For this review, use the dimensioned drawing (mm, ordinates from the lowest corner) and the shaded views. A direction names the side the tool comes from. Give positions to 0.01 mm unless a question says otherwise; leave off trailing zeros. Order: outer loops, then holes, each group sorted by start corner. A loop starts at its lowest first (then second) coordinate and runs counter-clockwise, first axis right, second up. Notation, with made-up numbers: M -24,-30.5 L 3,-30.5 A24 ccw 3,5.5 Z; hole C -27,0.25 d5. An arc over 180 degrees is marked long. Use CSV: the item, a comma, the result in double quotes. Start each with the question number.
(1) Consider section C-C (x = 21). Write out the cut boundary in (y, z).
(2) Consider section B-B (y = 15.5). Write out the cut boundary in (x, z), and give its area (3 significant figures).
(3) Wall thickness on L1, parallel to X at y = 16.4, z = 25; L2, parallel to Y at x = 36.5, z = 21.5; L3, parallel to Y at x = 21, z = 16.5: over which ranges is each line inside the solid? List them lowest first. Write a range as from..to.
(4) Tool access review of the marked faces 1, 2 and 3: name each direction out of +Z, -Z, +X, -X, +Y, -Y from which nothing blocks a thin tool from reaching the whole face with its end or side.
(5) Consider section A-A (z = 30). Write out the cut boundary in (x, y).
(6) Clearance check with flat-ended pins moving along their axes: P1, Ø4, axis at x = 14.5, z = 51.5, coming from the -Y side; P2, Ø1.5, axis at y = 9.5, z = 28, coming from the -X side; P3, Ø2, axis at x = 35.5, z = 35, coming from the +Y side. State where each tip first meets the part, or that it passes through.
(7) Consider section D-D (y = 5.25). Write out the cut boundary in (x, z).
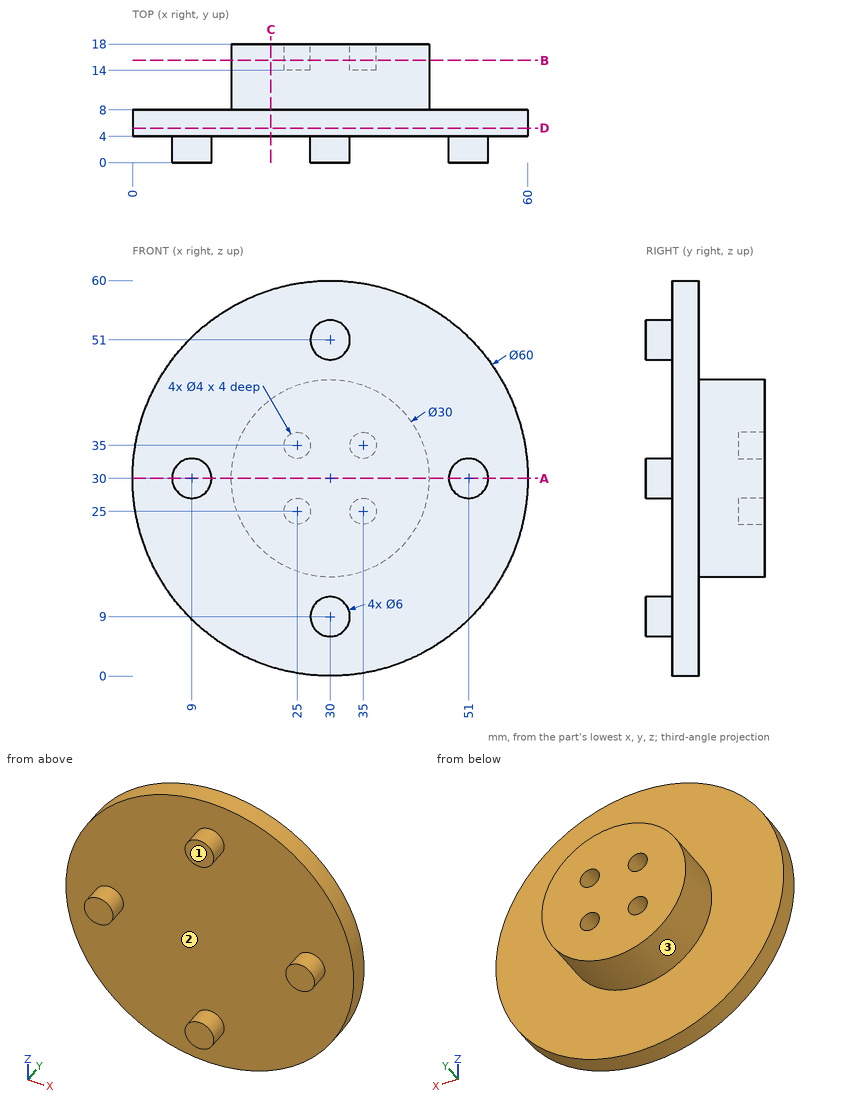
Check result:
1,outline,"M 4,1.38 L 8,1.38 L 8,18 L 18,18 L 18,42 L 8,42 L 8,58.62 L 4,58.62 Z"
2,outline,"C 30,30 d30; hole C 25,25 d4; hole C 25,35 d4; hole C 35,25 d4; hole C 35,35 d4"
2,area,"657 mm^2"
3,L1,"x = 15.86..23, 27..33, 37..44.14"
3,L2,"y = 4..18"
3,L3,"y = 4..8"
4,face 1,"+Z, -Z, +X, -X, -Y"
4,face 2,"-Y"
4,face 3,"+Y"
5,outline,"M 0,4 L 6,4 L 6,0 L 12,0 L 12,4 L 48,4 L 48,0 L 54,0 L 54,4 L 60,4 L 60,8 L 45,8 L 45,18 L 15,18 L 15,8 L 0,8 Z"
6,P1,"stops at y = 4"
6,P2,"stops at x = 15.05"
6,P3,"stops at y = 14"
7,outline,"C 30,30 d60"
